from build123d import *

# Parameters (mm, degrees)
F2_R     = 20
F3_DEPTH = 50
F4_W     = 62.4089296907
F4_H     = 39.0701051801
F5_DEPTH = 50


# Not quite as in the source:
# - a fillet or chamfer that OpenCascade refuses, or shapes differently, is made with other operations: its cross-section is extruded or revolved along the edge and cut away or added


with BuildPart() as f1:
    # F0 (on Top) → F1 (revolve)
    with BuildSketch(Plane.XY):
        with BuildLine():
            Line((0, 40), (0, -40))
            ThreePointArc((0, -40), (40, 0), (0, 40))
        make_face()
    revolve(axis=Axis((0, 0, 0), (0, -1, 0)))

    # F2 (on Right) → F3 (cut, symmetric)
    with BuildSketch(Plane.YZ):
        Circle(F2_R)
    extrude(amount=F3_DEPTH, both=True, mode=Mode.SUBTRACT)

    # F4 (on Right) → F5 (cut, symmetric)
    with BuildSketch(Plane.YZ):
        with Locations((0.7427642122, 53.4269148484)):
            Rectangle(F4_W, F4_H)
    extrude(amount=F5_DEPTH, both=True, mode=Mode.SUBTRACT)

    # F6: chamfer of 2 on 1 edges, made by hand

    # F6_s1 → F6_t2 (revolve, cut)
    with BuildSketch(Plane.YZ):
        with BuildLine():
            Line((23.2462048843, 32.5816827787), (19.0643837553, 33.916183436))
            Line((19.0643837553, 33.916183436), (19.0643837553, 33.956183436))
            ThreePointArc((19.0643837553, 33.956183436), (20.1545935913, 33.9318622583), (21.2448034273, 33.9318622583))
            Line((21.2448034273, 33.9318622583), (21.2660482307, 33.9257541206))
            ThreePointArc((21.2660482307, 33.9257541206), (22.2709130322, 33.2747356521), (23.2693748758, 32.6142887827))
            Line((23.2693748758, 32.6142887827), (23.2462048843, 32.5816827787))
        make_face()
    revolve(axis=Axis((0, 0, 33.8918622583), (0, 0, -1)), mode=Mode.SUBTRACT)


solid = f1.part
Can you work these out from the model? Positions are in its coordinate system, mm. Round coordinates to 2 decimals unless told otherwise and drop trailing zeros. Loops run counter-clockwise (first coordinate to the right, second up) from the corner with the lowest first, then second, coordinate; pieces in that order, holes last. Notation, with made-up numbers: (23, 23.25) - (47, 23.25) arc R21 cw to (47, 45.25) - close; hole circle Ø3 at (2.5, -1.5). An arc over 180 degrees is marked (long way). Write item = value, one per line. Start each with the question number.
(1) If we section it at A-A (y = 0): Please give me the cut outline in (x, z).
(2) If I drill on probe 1 along Y at (x, z) = (2, 0); probe 2 along Y at (x, z) = (5, 0); probe 3 along Z at (x, y) = (6, 0), over which ranges is the centre line in solid material (lowest first)? Write a range as [from, to].
(3) If we mould it in two halves opening along Y, with no side actions, what happens to faces 1 (the face through (-18.88, -4.19, 33.83)), 2 (the face through (0, 0, 33.892)), 3 (the face through (0.485, -4.336, -19.524))? For each: released by +Y, released by -Y, zero draft, split by the parting line, or undercut.
(4) If we section it at B-B (x = 0): Please give me the cut outline in (y, z).
(5) If we section it at D-D (z = 16): Please give me the cut outline in (x, y).
(6) If we section it at C-C (z = 0): Please give me the cut outline in (x, y), and give its area (3 significant figures).
(7) For P1, Ø3, axis at y = 31.5, z = 18.5, coming from the -X side; P2, Ø8, axis at y = -5.5, z = -29, coming from the +X side; P3, Ø5, axis at y = 23.5, z = -4.5, coming from the -X side; P4, Ø12, axis at y = 11.5, z = -21, coming from the +X side, each with a flat end and sliding along its axis, tell me the tip position at first contact or that it passes through.
Ans:
q1.outline = (-34.64, -20) arc R40 ccw to (34.64, -20) - close; (-34.64, 20) - (34.64, 20) arc R40 ccw to (23.17, 32.61) - (19.14, 33.89) - (-19.14, 33.89) - (-23.17, 32.61) arc R40 ccw to start
q2.probe_1 = [-39.95, -20], [20, 39.95]
q2.probe_2 = [-39.69, -20], [20, 39.69]
q2.probe_3 = [-39.55, -20], [20, 33.89]
q3.face_1 = split by the parting line
q3.face_2 = zero draft
q3.face_3 = undercut
q4.outline = (-23.17, 32.61) arc R40 ccw (long way) to (23.17, 32.61) - (19.14, 33.89) - (-19.14, 33.89) - close; hole circle Ø40 at (0, 0)
q5.outline = (-34.64, -12) arc R36.66 ccw to (34.64, -12) - close; (-34.64, 12) - (34.64, 12) arc R36.66 ccw to start
q6.outline = (-34.64, -20) arc R40 ccw to (34.64, -20) - close; (-34.64, 20) - (34.64, 20) arc R40 ccw to start
q6.area = 1,970 mm²
q7.P1 = -19.31
q7.P2 = 30.8
q7.P3 = -33.78
q7.P4 = 34.64
